CAD build for the part. Positions are in the model's coordinates, mm. Coordinates: 2 decimals unless noted, no trailing zeros. Order: outer loops, then holes, each group sorted by start corner. A loop starts at its lowest first (then second) coordinate and runs counter-clockwise, first axis right, second up. Notation, with made-up numbers: M 77,7 L 133,7 A8 cw 133,16 Z; hole C 66.5,63.25 d3. An arc over 180 degrees is marked long. Write item = value, one per line.
from build123d import *

# Parameters (mm, degrees)
BOSS_EXTRUDE4_START  = 175
SKETCH1_R            = 100
BOSS_EXTRUDE4_DEPTH  = 8
CUT_EXTRUDE5_DEPTH   = 10
SKETCH19_R           = 125
SKETCH19_R_2         = 100
BOSS_EXTRUDE11_DEPTH = 8
SKETCH20_R           = 1.7
CUT_EXTRUDE8_DEPTH   = 8
CUT_EXTRUDE9_START   = 183
SKETCH22_R           = 13
CUT_EXTRUDE9_DEPTH   = 8


with BuildPart() as part:
    # Sketch1 → Boss-Extrude4 (new body)
    with BuildSketch(Plane(origin=(0, 0, 0), x_dir=(1, 0, 0), z_dir=(0, 1, 0)).offset(BOSS_EXTRUDE4_START)):
        Circle(SKETCH1_R)
    extrude(amount=BOSS_EXTRUDE4_DEPTH)

    # Sketch15 → Cut-Extrude5 (cut)
    with BuildSketch(Plane(origin=(0, 183, 0), x_dir=(1, 0, 0), z_dir=(0, 1, 0))):
        with BuildLine():
            Line((1.7, 38.5), (1.7, 72))
            ThreePointArc((1.7, 72), (0, 73.7), (-1.7, 72))
            Line((-1.7, 72), (-1.7, 38.5))
            ThreePointArc((-1.7, 38.5), (0, 36.8), (1.7, 38.5))
        make_face()
        with BuildLine():
            Line((32.491978046, -20.722243186), (61.503829072, -37.472243186))
            ThreePointArc((61.503829072, -37.472243186), (63.826072259, -36.85), (63.203829072, -34.527756814))
            Line((63.203829072, -34.527756814), (34.191978046, -17.777756814))
            ThreePointArc((34.191978046, -17.777756814), (31.869734859, -18.4), (32.491978046, -20.722243186))
        make_face()
        with BuildLine():
            Line((-34.191978046, -17.777756814), (-63.203829072, -34.527756814))
            ThreePointArc((-63.203829072, -34.527756814), (-63.826072259, -36.85), (-61.503829072, -37.472243186))
            Line((-61.503829072, -37.472243186), (-32.491978046, -20.722243186))
            ThreePointArc((-32.491978046, -20.722243186), (-31.869734859, -18.4), (-34.191978046, -17.777756814))
        make_face()
    extrude(amount=-CUT_EXTRUDE5_DEPTH, mode=Mode.SUBTRACT)

    # Sketch19 → Boss-Extrude11 (add)
    with BuildSketch(Plane(origin=(0, 183, 0), x_dir=(1, 0, 0), z_dir=(0, 1, 0))):
        Circle(SKETCH19_R)
        Circle(SKETCH19_R_2, mode=Mode.SUBTRACT)
    extrude(amount=-BOSS_EXTRUDE11_DEPTH)

    # Sketch20 → Cut-Extrude8 (cut)
    with BuildSketch(Plane(origin=(0, 183, 0), x_dir=(1, 0, 0), z_dir=(0, 1, 0))):
        with Locations((30, -51.961524227)):
            Circle(SKETCH20_R)
        with Locations((40, -69.282032303)):
            Circle(SKETCH20_R)
        with Locations((20, -34.641016151)):
            Circle(SKETCH20_R)
        with Locations((-30, -51.961524227)):
            Circle(SKETCH20_R)
        with Locations((-40, -69.282032303)):
            Circle(SKETCH20_R)
        with Locations((-20, -34.641016151)):
            Circle(SKETCH20_R)
        with Locations((-60, 0)):
            Circle(SKETCH20_R)
        with Locations((-80, 0)):
            Circle(SKETCH20_R)
        with Locations((-40, 0)):
            Circle(SKETCH20_R)
        with Locations((-30, 51.961524227)):
            Circle(SKETCH20_R)
        with Locations((-40, 69.282032303)):
            Circle(SKETCH20_R)
        with Locations((-20, 34.641016151)):
            Circle(SKETCH20_R)
        with Locations((30, 51.961524227)):
            Circle(SKETCH20_R)
        with Locations((40, 69.282032303)):
            Circle(SKETCH20_R)
        with Locations((20, 34.641016151)):
            Circle(SKETCH20_R)
        with Locations((60, 0)):
            Circle(SKETCH20_R)
        with Locations((80, 0)):
            Circle(SKETCH20_R)
        with Locations((40, 0)):
            Circle(SKETCH20_R)
        with BuildLine():
            ThreePointArc((-21.032101141, 108.489004544), (-55.220471881, 95.723105208), (-83.386729073, 72.51804465))
            ThreePointArc((-83.386729073, 72.51804465), (-82.353167452, 57.69222173), (-67.527344531, 58.725783351))
            ThreePointArc((-67.527344531, 58.725783351), (-44.718048919, 77.517456037), (-17.031990051, 87.855399404))
            ThreePointArc((-17.031990051, 87.855399404), (-8.715243026, 100.172257519), (-21.032101141, 108.489004544))
        make_face()
        with BuildLine():
            ThreePointArc((83.438183396, 72.458836155), (55.288404899, 95.683884061), (21.109104364, 108.47404804))
            ThreePointArc((21.109104364, 108.47404804), (8.786345893, 100.16604596), (17.094347973, 87.84328749))
            ThreePointArc((17.094347973, 87.84328749), (44.773061705, 77.48569439), (67.569012718, 58.677835764))
            ThreePointArc((67.569012718, 58.677835764), (82.394098253, 57.633750621), (83.438183396, 72.458836155))
        make_face()
        with BuildLine():
            ThreePointArc((104.470284537, -36.030168389), (110.508876779, -0.039221146), (104.495833436, 35.95600339))
            ThreePointArc((104.495833436, 35.95600339), (91.139513345, 42.47382423), (84.621692504, 29.117504139))
            ThreePointArc((84.621692504, 29.117504139), (89.491110624, -0.031761647), (84.601002769, -29.177563641))
            ThreePointArc((84.601002769, -29.177563641), (91.109341279, -42.538506898), (104.470284537, -36.030168389))
        make_face()
        with BuildLine():
            ThreePointArc((21.032101141, -108.489004544), (55.220471881, -95.723105208), (83.386729073, -72.51804465))
            ThreePointArc((83.386729073, -72.51804465), (82.353167452, -57.69222173), (67.527344531, -58.725783351))
            ThreePointArc((67.527344531, -58.725783351), (44.718048919, -77.517456037), (17.031990051, -87.855399404))
            ThreePointArc((17.031990051, -87.855399404), (8.715243026, -100.172257519), (21.032101141, -108.489004544))
        make_face()
        with BuildLine():
            ThreePointArc((-83.438183396, -72.458836155), (-55.288404899, -95.683884061), (-21.109104364, -108.47404804))
            ThreePointArc((-21.109104364, -108.47404804), (-8.786345893, -100.16604596), (-17.094347973, -87.84328749))
            ThreePointArc((-17.094347973, -87.84328749), (-44.773061705, -77.48569439), (-67.569012718, -58.677835764))
            ThreePointArc((-67.569012718, -58.677835764), (-82.394098253, -57.633750621), (-83.438183396, -72.458836155))
        make_face()
        with BuildLine():
            ThreePointArc((-104.470284537, 36.030168389), (-110.508876779, 0.039221146), (-104.495833436, -35.95600339))
            ThreePointArc((-104.495833436, -35.95600339), (-91.139513345, -42.47382423), (-84.621692504, -29.117504139))
            ThreePointArc((-84.621692504, -29.117504139), (-89.491110624, 0.031761647), (-84.601002769, 29.177563641))
            ThreePointArc((-84.601002769, 29.177563641), (-91.109341279, 42.538506898), (-104.470284537, 36.030168389))
        make_face()
    extrude(amount=-CUT_EXTRUDE8_DEPTH, mode=Mode.SUBTRACT)

    # Sketch22 → Cut-Extrude9 (cut)
    with BuildSketch(Plane(origin=(0, 0, 0), x_dir=(1, 0, 0), z_dir=(0, 1, 0)).offset(CUT_EXTRUDE9_START)):
        with Locations((23.034671131, 13.299073578)):
            Circle(SKETCH22_R)
        with Locations((0, -26.598147157)):
            Circle(SKETCH22_R)
        with Locations((-23.034671131, 13.299073578)):
            Circle(SKETCH22_R)
    extrude(amount=-CUT_EXTRUDE9_DEPTH, mode=Mode.SUBTRACT)


solid = part.part
(1) Slice it at C-C, the plane y = 180.5. State how many separate pieces and enclosed holes the cut face has, then the cut area to 3 significant figures.
Evaluation:
separate_pieces = 1
enclosed_holes = 30
area = 36,500 mm²
(2) Slice it at A-A, the plane z = -104. Write the cut outline in (x, y).
Evaluation:
outline = M -69.35,175 L -37.37,175 L -37.37,183 L -69.35,183 Z; M -10.29,175 L 10.37,175 L 10.37,183 L -10.29,183 Z; M 37.37,175 L 69.35,175 L 69.35,183 L 37.37,183 Z
(3) Wall check: line 1 (Z direction, x = 60, y = 180.5); line 2 (X direction, y = 180, z = -75.5); line 3 (Z direction, x = 74, y = 182.5). Give the ranges that are in metal, low to high. Write a range as from..to.
Evaluation:
line_1 = -109.66..-92.8, -66.4..-1.7, 1.7..32.68, 36.6..66.4, 92.8..109.66
line_2 = -99.62..-80.7, -48.05..48.05, 80.7..99.62
line_3 = -100.74..-82.07, -55.17..55.21, 82.07..100.74
(4) Slice it at B-B, the plane x = -95.5. Write the cut outline in (y, z), then the cut area to 3 significant figures.
Evaluation:
outline = M 175,-80.65 L 183,-80.65 L 183,-43.07 L 175,-43.07 Z; M 175,43 L 183,43 L 183,80.65 L 175,80.65 Z
area = 602 mm²
(5) Pin check, flat tips, straight feed: pin 1 Ø4 at (y, z) = (180.5, -5.5) entering from -X; pin 2 Ø4 at (x, y) = (-21, 180.5) entering from +Z; pin 3 Ø4 at (y, z) = (181.5, -87) entering from -X. Stop position of each tip, or through.
Evaluation:
pin_1 = -124.95
pin_2 = 123.55
pin_3 = -91.65
